Input: part model. Units: mm. Frame: model coordinates. A direction names the side the tool comes from. Round coordinates to 2 decimals unless told otherwise and drop trailing zeros. Loops run counter-clockwise (first coordinate to the right, second up) from the corner with the lowest first, then second, coordinate; pieces in that order, holes last. Notation, with made-up numbers: M -12.5,88.5 L 13.5,88.5 A20 cw 13.5,120.5 Z; hole C 7,45.5 d3. An arc over 180 degrees is marked long. Return JSON: item names as keys, results as strings. Group by question number.
1) Section A-A (z = 91.5). Output: boundary loops of the cut face in (x, y).
2) Mould query, pull axis Z, two halves, no side actions, for faces 1 (the face through (-3, 0, -3)), 2 (the face through (-3, 6, -200)), 3 (the face through (-200, 6, -145.6)). Classes: +Z half, -Z half, draft (parallel to the pull), parting line (faces both ways), or undercut.
3) Access query for faces 4 (the face through (-150, 6, 1)), 5 (the face through (-250, 6, 3)). Directions: +Z, -Z, +X, -X, +Y, -Y. A direction counts if a zero-diameter tool reaches every point of the face in a straight line with its end or side. Return the directions, or none.
4) Material intervals for line 1 (X direction, y = 1.5, z = 78.5); line 2 (Z direction, x = 190, y = 7); line 3 (Z direction, x = 152.5, y = 11), sorted ascending. Write a range as from..to.
from build123d import *

# Parameters (mm, degrees)
SKETCH1_W                                  = 500
SKETCH1_H                                  = 400
BOSS_EXTRUDE1_DEPTH                        = 12
SKETCH2_W                                  = 4.4
SKETCH2_H                                  = 200
CUT_EXTRUDE1_DEPTH                         = 12
SKETCH5_W                                  = 50
SKETCH5_H                                  = 4.4
CUT_EXTRUDE2_DEPTH                         = 12
MIRROR5_AT_THE_SECOND_PLANE_COPY_1_SKETC_W = 50
MIRROR5_AT_THE_SECOND_PLANE_COPY_1_SKETC_H = 4.4
MIRROR5_AT_THE_SECOND_PLANE_COPY_1_DEPTH   = 12


with BuildPart() as part:
    # Sketch1 → Boss-Extrude1 (new body)
    with BuildSketch(Plane(origin=(0, 0, 0), x_dir=(1, 0, 0), z_dir=(0, 1, 0))):
        Rectangle(SKETCH1_W, SKETCH1_H)
    extrude(amount=BOSS_EXTRUDE1_DEPTH)

    # Sketch2 → Cut-Extrude1 (cut)
    with BuildSketch(Plane(origin=(0, 12, 0), x_dir=(1, 0, 0), z_dir=(0, 1, 0))):
        with Locations((-152.2, 0)):
            Rectangle(SKETCH2_W, SKETCH2_H)
    cut_extrude1 = extrude(amount=-CUT_EXTRUDE1_DEPTH, mode=Mode.SUBTRACT)

    # Mirror2: Cut-Extrude1 across plane
    add(cut_extrude1.mirror(Plane(origin=(0, 0, 0), x_dir=(0, 0, 1), z_dir=(1, 0, 0))), mode=Mode.SUBTRACT)

    # Sketch5 → Cut-Extrude2 (cut)
    with BuildSketch(Plane(origin=(0, 12, 0), x_dir=(1, 0, 0), z_dir=(0, 1, 0))):
        with Locations((-199.9, 147.8)):
            Rectangle(SKETCH5_W, SKETCH5_H)
    cut_extrude2 = extrude(amount=-CUT_EXTRUDE2_DEPTH, mode=Mode.SUBTRACT)

    # Mirror5: Cut-Extrude2 across plane
    add(cut_extrude2.mirror(Plane.XY), mode=Mode.SUBTRACT)

    # Mirror5 at the second plane: Cut-Extrude2 across plane
    add(cut_extrude2.mirror(Plane(origin=(0, 0, 0), x_dir=(0, 0, 1), z_dir=(1, 0, 0))), mode=Mode.SUBTRACT)

    # Mirror5 at the second plane copy 1 sketc → Mirror5 at the second plane copy 1 (cut)
    with BuildSketch(Plane(origin=(0, 12, 0), x_dir=(-1, 0, 0), z_dir=(0, 1, 0))):
        with Locations((-199.9, 147.8)):
            Rectangle(MIRROR5_AT_THE_SECOND_PLANE_COPY_1_SKETC_W, MIRROR5_AT_THE_SECOND_PLANE_COPY_1_SKETC_H)
    extrude(amount=-MIRROR5_AT_THE_SECOND_PLANE_COPY_1_DEPTH, mode=Mode.SUBTRACT)


solid = part.part
Returned:
{
 "1": {"outline": "M -250,0 L -154.4,0 L -154.4,12 L -250,12 Z; M -150,0 L 150,0 L 150,12 L -150,12 Z; M 154.4,0 L 250,0 L 250,12 L 154.4,12 Z"},
 "2": {"face 1": "draft", "face 2": "-Z half", "face 3": "undercut"},
 "3": {"face 4": "+Y, -Y", "face 5": "+Z, -Z, -X, +Y, -Y"},
 "4": {"line 1": "x = -250..-154.4, -150..150, 154.4..250", "line 2": "z = -200..-150, -145.6..145.6, 150..200", "line 3": "z = -200..-100, 100..200"}
}
